from build123d import *

# Parameters (mm, degrees)
SKETCH2_R          = 4.45
CUT_EXTRUDE1_DEPTH = 7
SKETCH3_R          = 1.1
CUT_EXTRUDE2_DEPTH = 18.866890468
SKETCH4_R          = 2.5
CUT_EXTRUDE3_DEPTH = 14.86689


with BuildPart() as part:
    # Sketch1 → Revolve1 (revolve)
    with BuildSketch(Plane(origin=(0, 0, 0), x_dir=(1, 0, 0), z_dir=(0, 1, 0))):
        Polygon((10.193859716, 12.315), (10.193859716, 7), (14.693859716, 7), (14.693859716, 5), (16.193859716, 5), (16.193859716, 0), (-7.673030752, 0), (-7.673030752, 14.5), (7.437816357, 13.69), align=None)
    revolve(axis=Axis((-18.233766234, 0, 0), (1, 0, 0)))

    # Sketch2 → Cut-Extrude1 (cut)
    with BuildSketch(Plane.ZY.offset(7.673030752)):
        Circle(SKETCH2_R)
    extrude(amount=-CUT_EXTRUDE1_DEPTH, mode=Mode.SUBTRACT)

    # Sketch3 → Cut-Extrude2 (cut, through all)
    with BuildSketch(Plane(origin=(10.193859716, 0, 0), x_dir=(0, 0, -1), z_dir=(1, 0, 0))):
        with Locations((0, 10)):
            Circle(SKETCH3_R)
        with Locations((7.071067812, 7.071067812)):
            Circle(SKETCH3_R)
        with Locations((10, 0)):
            Circle(SKETCH3_R)
        with Locations((7.071067812, -7.071067812)):
            Circle(SKETCH3_R)
        with Locations((0, -10)):
            Circle(SKETCH3_R)
        with Locations((-7.071067812, -7.071067812)):
            Circle(SKETCH3_R)
        with Locations((-10, 0)):
            Circle(SKETCH3_R)
        with Locations((-7.071067812, 7.071067812)):
            Circle(SKETCH3_R)
    extrude(amount=-CUT_EXTRUDE2_DEPTH, mode=Mode.SUBTRACT)

    # Sketch4 → Cut-Extrude3 (cut)
    with BuildSketch(Plane.ZY.offset(7.673030752)):
        with Locations((0, 10)):
            Circle(SKETCH4_R)
        with Locations((7.071067812, 7.071067812)):
            Circle(SKETCH4_R)
        with Locations((10, 0)):
            Circle(SKETCH4_R)
        with Locations((7.071067812, -7.071067812)):
            Circle(SKETCH4_R)
        with Locations((0, -10)):
            Circle(SKETCH4_R)
        with Locations((-7.071067812, -7.071067812)):
            Circle(SKETCH4_R)
        with Locations((-10, 0)):
            Circle(SKETCH4_R)
        with Locations((-7.071067812, 7.071067812)):
            Circle(SKETCH4_R)
    extrude(amount=-CUT_EXTRUDE3_DEPTH, mode=Mode.SUBTRACT)


solid = part.part
Work out the finished part from the listing and answer in its coordinate system (mm). A direction names the side the tool comes from. Coordinates: 2 decimals unless noted, no trailing zeros. Answer in a Markdown table with one row per item. Add a question column.
1. The mould has two halves that part along Y. Classify faces 4 (the flat face through (14.694, 5, 2)), 5 (the cylindrical face through (15.45, -4.88, 1.08)), 6 (the cylindrical face through (8.715, 8.926, 0.238)), 7 (the cylindrical face through (8.715, -0.421, -11.016)): pulls with the +Y half, pulls with the -Y half, needs draft (parallel to the pull), parting line crosses it, or undercut.
2. Find section A-A, the plane z = 0. State how many separate pieces and enclosed holes the cut face has, then the cut area to 3 significant figures.
3. Consider L1, parallel to Z at x = 7.5, y = 8; L2, parallel to Y at x = 4, z = -7.75; L3, parallel to Z at x = 7.5, y = 7.75. Determine where each line is inside the solid, lowest interval first.
4. Flat-ended cylindrical pins translate along their axes: P1, Ø10, axis at y = 1, z = -1.5, coming from the -X side; P2, Ø3, axis at x = 2, z = 6, coming from the +Y side; P3, Ø4, axis at x = 7.5, y = -0.5, coming from the +Z side; P4, Ø3, axis at y = -10, z = 0, coming from the +X side. Find the tip coordinate at first contact, or state that the pin passes through.
5. A tool of negligible diameter and unlimited length cuts with its end or side. For faces 1 (the cylindrical face through (-0.34, -6.96, -9.57)), 2 (the flat face through (10.194, -5.3, -5.3)), 3 (the flat face through (-7.673, 3.4, -3.4)), from which of +Z, -Z, +X, -X, +Y, -Y can it reach the whole face along a straight path? Write none if from no direction.
Reported:
| question | item | result |
|---|---|---|
| 1 | face 4 | needs draft |
| 1 | face 5 | parting line crosses it |
| 1 | face 6 | undercut |
| 1 | face 7 | undercut |
| 2 | separate pieces | 3 |
| 2 | enclosed holes | 0 |
| 2 | area | 351 mm^2 |
| 3 | L1 | z = -11.07 to -7.66, -6.48 to 6.48, 7.66 to 11.07 |
| 3 | L2 | y = -11.51 to -9.48, -4.67 to -1.09, 1.09 to 4.67, 9.48 to 11.51 |
| 3 | L3 | z = -11.25 to -7.94, -6.21 to 6.21, 7.94 to 11.25 |
| 4 | P1 | stops at x = -7.67 |
| 4 | P2 | stops at y = 13.24 |
| 4 | P3 | stops at z = 13.79 |
| 4 | P4 | stops at x = 10.19 |
| 5 | face 1 | -X |
| 5 | face 2 | +X |
| 5 | face 3 | +Z, -Z, -X, +Y, -Y |
